Geometry check sheet. Reference: drawing and pictorial views, mm from the part's lowest x, y, z. A direction names the side the tool comes from. Coordinates: 2 decimals unless noted, no trailing zeros. Loops run counter-clockwise (first coordinate to the right, second up) from the corner with the lowest first, then second, coordinate; pieces in that order, holes last. Notation, with made-up numbers: (27, 62) -> (84, 62) arc R24 cw to (84, 73) -> close; hole circle Ø1 at (-8.5, 16). An arc over 180 degrees is marked (long way). Answer as a JSON object with one key per item and string values.
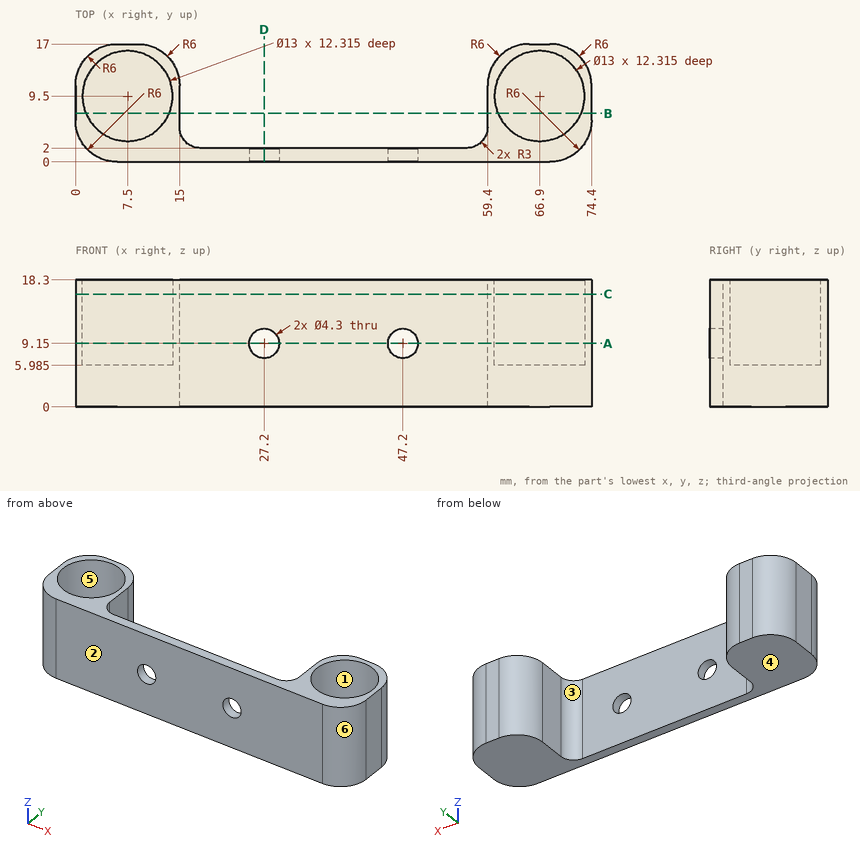
1. Section check B-B, the plane y = 7. Record the boundary of the cut face in (x, z) (3 decimals), then the cut area to 3 significant figures.
Evaluation:
{"outline": "(0, 0) -> (15, 0) -> (15, 18.3) -> (13.5, 18.3) -> (13.5, 5.985) -> (1.5, 5.985) -> (1.5, 18.3) -> (0, 18.3) -> close; (59.4, 0) -> (74.4, 0) -> (74.4, 18.3) -> (72.9, 18.3) -> (72.9, 5.985) -> (60.9, 5.985) -> (60.9, 18.3) -> (59.4, 18.3) -> close", "area": "253 mm^2"}
2. Depth check by flat-ended pin: P1, Ø2.5, axis at x = 27.2, z = 9.15, coming from the +Y side; P2, Ø4, axis at x = 50.5, z = 9, coming from the +Y side. Enter the tip coordinate at first touch or a pass-through.
Evaluation:
{"P1": "passes through", "P2": "stops at y = 2"}
3. Section check C-C, the plane z = 16.25. Record the boundary of the cut face in (x, y), then the cut area to 3 significant figures.
Evaluation:
{"outline": "(0, 6) arc R6 ccw to (6, 0) -> (68.4, 0) arc R6 ccw to (74.4, 6) -> (74.4, 11) arc R6 ccw to (68.4, 17) -> (65.4, 17) arc R6 ccw to (59.4, 11) -> (59.4, 5) arc R3 cw to (56.4, 2) -> (18, 2) arc R3 cw to (15, 5) -> (15, 11) arc R6 ccw to (9, 17) -> (6, 17) arc R6 ccw to (0, 11) -> close; hole circle Ø13 at (7.5, 9.5); hole circle Ø13 at (66.9, 9.5)", "area": "291 mm^2"}
4. Tool access check on the marked faces 1, 2 and 3. Record the directions out of +Z, -Z, +X, -X, +Y, -Y that give a thin tool (end or side, any length) a straight path to the whole face; none if there is none.
Evaluation:
{"face 1": "+Z", "face 2": "+Z, -Z, +X, -X, -Y", "face 3": "+Z, -Z, +Y"}
5. Section check D-D, the plane x = 27.2. Record the boundary of the cut face in (y, z), then the cut area to 3 significant figures.
Evaluation:
{"outline": "(0, 0) -> (2, 0) -> (2, 7) -> (0, 7) -> close; (0, 11.3) -> (2, 11.3) -> (2, 18.3) -> (0, 18.3) -> close", "area": "28.0 mm^2"}
6. Mould release check, pull along X, two halves, no side actions. Record for the marked faces 4, 5 and 6: released by +X, released by -X, zero draft, split by the parting line, or undercut.
Evaluation:
{"face 4": "zero draft", "face 5": "undercut", "face 6": "released by +X"}
7. Thickness scan on probe 1 along X at (y, z) = (15.5, 16.75); probe 2 along X at (y, z) = (11, 5); probe 3 along X at (y, z) = (5.75, 14.75). Record the ranges inside material, lowest first. Write a range as from..to.
Evaluation:
{"probe 1": "x = 2.03..5, 10..12.97, 61.43..64.4, 69.4..72.37", "probe 2": "x = 0..15, 59.4..74.4", "probe 3": "x = 0.01..2.19, 12.81..15, 59.4..61.59, 72.21..74.39"}
8. Section check A-A, the plane z = 9.15. Record the boundary of the cut face in (x, y), then the cut area to 3 significant figures.
Evaluation:
{"outline": "(0, 6) arc R6 ccw to (6, 0) -> (25.05, 0) -> (25.05, 2) -> (18, 2) arc R3 cw to (15, 5) -> (15, 11) arc R6 ccw to (9, 17) -> (6, 17) arc R6 ccw to (0, 11) -> close; (29.35, 0) -> (45.05, 0) -> (45.05, 2) -> (29.35, 2) -> close; (49.35, 0) -> (68.4, 0) arc R6 ccw to (74.4, 6) -> (74.4, 11) arc R6 ccw to (68.4, 17) -> (65.4, 17) arc R6 ccw to (59.4, 11) -> (59.4, 5) arc R3 cw to (56.4, 2) -> (49.35, 2) -> close; hole circle Ø13 at (7.5, 9.5); hole circle Ø13 at (66.9, 9.5)", "area": "274 mm^2"}
